from build123d import *

# Parameters (mm, degrees)
EXTRUDE_2_DEPTH           = 2
HOLE_WIZARD_0_D           = 2.8
HOLE_WIZARD_0_DEPTH       = 10.1
HOLE_WIZARD_0_CSINK_D     = 4.8
HOLE_WIZARD_0_CSINK_ANGLE = 90
HOLE_WIZARD_0_TIP         = 0.841204867
SKETCH_7_R                = 5.75
SKETCH_7_R_2              = 4.25
EXTRUDE_1_DEPTH           = 0.5


with BuildPart() as part:
    # 草图3 → 凸台-拉伸2 (new body)
    with BuildSketch(Plane.XY):
        with BuildLine():
            Line((10, -28), (-10, -28))
            ThreePointArc((-10, -28), (-38, 0), (-10, 28))
            Line((-10, 28), (10, 28))
            ThreePointArc((10, 28), (38, 0), (10, -28))
        make_face()
    extrude(amount=EXTRUDE_2_DEPTH)

    # 打孔尺寸(%根据十字)槽沉头自攻螺钉的类型0
    with Locations(Plane.XY.offset(2)):
        with Locations((-29, 16), (-29, -16), (29, 16), (29, -16)):
            CounterSinkHole(HOLE_WIZARD_0_D / 2, HOLE_WIZARD_0_CSINK_D / 2, depth=HOLE_WIZARD_0_DEPTH, counter_sink_angle=HOLE_WIZARD_0_CSINK_ANGLE)
            with Locations((0, 0, -(HOLE_WIZARD_0_DEPTH + HOLE_WIZARD_0_TIP / 2))):  # 118° drill point
                Cone(0, HOLE_WIZARD_0_D / 2, HOLE_WIZARD_0_TIP, mode=Mode.SUBTRACT)

    # 草图7 → 拉伸-薄壁1 (add)
    # profile 1 of 4: a face of its own
    with BuildSketch(Plane.XY.offset(2)):
        with Locations((-30.673237657, 7.524443153)):
            Circle(SKETCH_7_R)
        with Locations((-30.673237657, 7.524443153)):
            Circle(SKETCH_7_R_2, mode=Mode.SUBTRACT)
    # profile 2 of 4: a face of its own
    with BuildSketch(Plane.XY.offset(2)):
        with Locations((-30.673237657, -7.524443153)):
            Circle(SKETCH_7_R)
        with Locations((-30.673237657, -7.524443153)):
            Circle(SKETCH_7_R_2, mode=Mode.SUBTRACT)
    # profile 3 of 4: a face of its own
    with BuildSketch(Plane.XY.offset(2)):
        with Locations((21, -19.052558883)):
            Circle(SKETCH_7_R)
        with Locations((21, -19.052558883)):
            Circle(SKETCH_7_R_2, mode=Mode.SUBTRACT)
    # profile 4 of 4: a face of its own
    with BuildSketch(Plane.XY.offset(2)):
        with Locations((21, 19.052558883)):
            Circle(SKETCH_7_R)
        with Locations((21, 19.052558883)):
            Circle(SKETCH_7_R_2, mode=Mode.SUBTRACT)
    extrude(amount=EXTRUDE_1_DEPTH)


solid = part.part
Could you check a few things on this model? Use its own coordinates, in mm. A direction names the side the tool comes from. Round coordinates to 2 decimals unless told otherwise and drop trailing zeros. Order: outer loops, then holes, each group sorted by start corner. A loop starts at its lowest first (then second) coordinate and runs counter-clockwise, first axis right, second up.
(1) Imagine slicing it at B-B (x = 29). Write out the boundary of the cut face in (y, z), plus the area to 3 significant figures.
Response values:
outline: (-20.57, 0) - (-17.4, 0) - (-17.4, 1) - (-18.4, 2) - (-20.57, 2) - close; (-14.6, 0) - (14.6, 0) - (14.6, 1) - (13.6, 2) - (-13.6, 2) - (-14.6, 1) - close; (17.4, 0) - (20.57, 0) - (20.57, 2) - (18.4, 2) - (17.4, 1) - close
area: 69.1 mm2
(2) If we mould it in two halves opening along X, with no side actions, what happens to faces 3 (the cylindrical face through (-37.993, -0.616, 0.986)), 4 (the flat face through (-31, 8, 2)), 5 (the flat face through (19, 15, 2.5))? For each: released by +X, released by -X, zero draft, split by the parting line, or undercut.
Response values:
face 3: released by -X
face 4: undercut
face 5: zero draft
(3) Imagine slicing it at A-A (z = 0.45). Write out the boundary of the cut face in (x, y).
Response values:
outline: (-10, -28) - (10, -28) arc R28 ccw to (10, 28) - (-10, 28) arc R28 ccw to start; hole circle Ø2.8 at (-29, -16); hole circle Ø2.8 at (-29, 16); hole circle Ø2.8 at (29, -16); hole circle Ø2.8 at (29, 16)
(4) Imagine slicing it at D-D (y = -22). Write out the boundary of the cut face in (x, z).
Response values:
outline: (-27.32, 0) - (27.32, 0) - (27.32, 2) - (25.94, 2) - (25.94, 2.5) - (24.06, 2.5) - (24.06, 2) - (17.94, 2) - (17.94, 2.5) - (16.06, 2.5) - (16.06, 2) - (-27.32, 2) - close
(5) Imagine slicing it at C-C (y = -16). Write out the boundary of the cut face in (x, z), plus the area to 3 significant figures.
Response values:
outline: (-32.98, 0) - (-30.4, 0) - (-30.4, 1) - (-31.4, 2) - (-32.98, 2) - close; (-27.6, 0) - (27.6, 0) - (27.6, 1) - (26.6, 2) - (25.87, 2) - (25.87, 2.5) - (23.96, 2.5) - (23.96, 2) - (18.04, 2) - (18.04, 2.5) - (16.13, 2.5) - (16.13, 2) - (-26.6, 2) - (-27.6, 1) - close; (30.4, 0) - (32.98, 0) - (32.98, 2) - (31.4, 2) - (30.4, 1) - close
area: 121 mm2
(6) Please list where these lines run through material, in increasing order: line 1 along Y through (x, z) = (21, 2.4); line 2 along Y through (x, z) = (-32.5, 2.4); line 3 along X through (y, z) = (-15, 0.55).
Response values:
line 1: y = -24.8 to -23.3, -14.8 to -13.3, 13.3 to 14.8, 23.3 to 24.8
line 2: y = -12.98 to -11.36, -3.69 to -2.07, 2.07 to 3.69, 11.36 to 12.98
line 3: x = -33.64 to -29.98, -28.02 to 28.02, 29.98 to 33.64
(7) I'm going to push flat-ended pins straight in: pin 1 (2.5 mm diameter, centred on x = 22.5, y = -20, fed in from +Z); pin 2 (1 mm diameter, centred on x = -27, z = 0.5, fed in from +Y); pin 3 (1.5 mm diameter, centred on x = 18.5, z = 1, fed in from +Y). Where does each tip first touch, or does it pass through?
Response values:
pin 1: stops at z = 2
pin 2: stops at y = 22.62
pin 3: stops at y = 26.91
(8) Which directions (+Z, -Z, +X, -X, +Y, -Y) give clear straight access to the entire face, cutting with the end or side of a thin tool? Please do faces 1 (the cylindrical face through (30.03, -15.05, 0.49)), 2 (the flat face through (21, -19, 2)).
Response values:
face 1: +Z, -Z
face 2: +Z
